Can you work these out from the model? Positions are in its coordinate system, mm. Face numbers are marked on the shaded views. A direction names the side the tool comes from. Give positions to 0.01 mm unless a question says otherwise; leave off trailing zeros. Order: outer loops, then holes, each group sorted by start corner. A loop starts at its lowest first (then second) coordinate and runs counter-clockwise, first axis right, second up. Notation, with made-up numbers: (46, -26.5) - (102, -26.5) arc R9 cw to (102, -11.5) - close; hole circle Ø8 at (18, 48.25). An arc over 180 degrees is marked (long way). Answer as a JSON object with one key per item and string values.
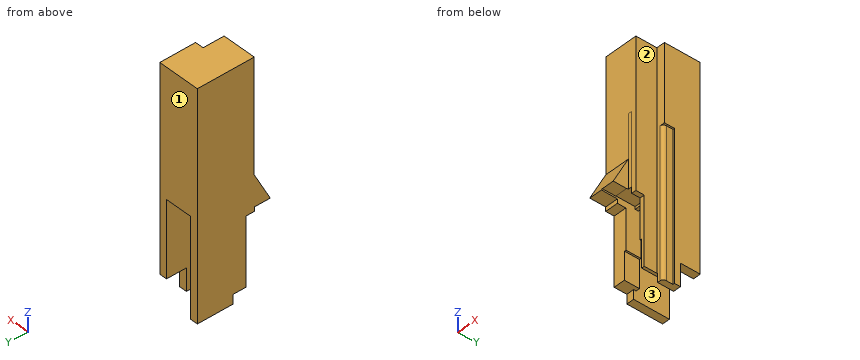
```python
from build123d import *

# Parameters (mm, degrees)
SKETCH1_W           = 50
SKETCH1_H           = 86.52
BOSS_EXTRUDE1_DEPTH = 266.658
SKETCH2_W           = 32
SKETCH2_H           = 116.66
CUT_EXTRUDE1_DEPTH  = 39.55
SKETCH3_W           = 32
SKETCH3_H           = 11
CUT_EXTRUDE2_DEPTH  = 276.341006506
SKETCH4_W           = 23
SKETCH4_H           = 33
CUT_EXTRUDE3_DEPTH  = 276.341006506
SKETCH5_W           = 19
SKETCH5_H           = 52
CUT_EXTRUDE4_DEPTH  = 276.341006506
SKETCH6_W           = 19
SKETCH6_H           = 3
CUT_EXTRUDE5_DEPTH  = 3
SKETCH7_W           = 26.66
SKETCH7_H           = 23.55
CUT_EXTRUDE6_DEPTH  = 11
SKETCH8_W           = 96.66
SKETCH8_H           = 18.97
CUT_EXTRUDE7_DEPTH  = 285.76692112
SKETCH9_W           = 80.656
SKETCH9_H           = 10
CUT_EXTRUDE8_DEPTH  = 285.76692112
SKETCH10_W          = 11
SKETCH10_H          = 25
CUT_EXTRUDE9_DEPTH  = 285.76692112
SKETCH11_W          = 175.66
SKETCH11_H          = 55.97
CUT_EXTRUDE10_DEPTH = 2
SKETCH12_W          = 266.658
SKETCH12_H          = 59.418393815
CUT_EXTRUDE11_DEPTH = 10
FILLET2_R           = 4
SKETCH13_W          = 19
SKETCH13_H          = 48.117373491
CUT_EXTRUDE12_DEPTH = 2.659
SKETCH16_W          = 19
SKETCH16_H          = 23.032
CUT_EXTRUDE13_DEPTH = 0.341
CUT_EXTRUDE14_DEPTH = 284.182272334
CUT_EXTRUDE15_DEPTH = 10
SKETCH22_W          = 5.5
SKETCH22_H          = 5.004
CUT_EXTRUDE16_DEPTH = 0.03
SKETCH24_W          = 4.5
SKETCH24_H          = 85.486763268
BOSS_EXTRUDE2_DEPTH = 0.03


with BuildPart() as part:
    # Sketch1 → Boss-Extrude1 (new body)
    with BuildSketch(Plane.XY):
        with Locations((-25, 43.26)):
            Rectangle(SKETCH1_W, SKETCH1_H)
    extrude(amount=BOSS_EXTRUDE1_DEPTH)

    # Sketch2 → Cut-Extrude1 (cut)
    with BuildSketch(Plane(origin=(0, 86.52, 0), x_dir=(1, 0, 0), z_dir=(0, 1, 0))):
        with Locations((-25, -58.33)):
            Rectangle(SKETCH2_W, SKETCH2_H)
    extrude(amount=-CUT_EXTRUDE1_DEPTH, mode=Mode.SUBTRACT)

    # Sketch3 → Cut-Extrude2 (cut, through all)
    with BuildSketch(Plane(origin=(0, 46.97, 0), x_dir=(1, 0, 0), z_dir=(0, 1, 0))):
        with Locations((-25, -5.5)):
            Rectangle(SKETCH3_W, SKETCH3_H)
    extrude(amount=-CUT_EXTRUDE2_DEPTH, mode=Mode.SUBTRACT)

    # Sketch4 → Cut-Extrude3 (cut, through all)
    with BuildSketch(Plane(origin=(0, 46.97, 0), x_dir=(1, 0, 0), z_dir=(0, 1, 0))):
        with Locations((-25, -27.5)):
            Rectangle(SKETCH4_W, SKETCH4_H)
    extrude(amount=-CUT_EXTRUDE3_DEPTH, mode=Mode.SUBTRACT)

    # Sketch5 → Cut-Extrude4 (cut, through all)
    with BuildSketch(Plane(origin=(0, 46.97, 0), x_dir=(1, 0, 0), z_dir=(0, 1, 0))):
        with Locations((-25, -70)):
            Rectangle(SKETCH5_W, SKETCH5_H)
    extrude(amount=-CUT_EXTRUDE4_DEPTH, mode=Mode.SUBTRACT)

    # Sketch6 → Cut-Extrude5 (cut)
    with BuildSketch(Plane(origin=(0, 46.97, 0), x_dir=(1, 0, 0), z_dir=(0, 1, 0))):
        with Locations((-25, -97.5)):
            Rectangle(SKETCH6_W, SKETCH6_H)
    extrude(amount=-CUT_EXTRUDE5_DEPTH, mode=Mode.SUBTRACT)

    # Sketch7 → Cut-Extrude6 (cut)
    with BuildSketch(Plane(origin=(0, 0, 0), x_dir=(0, 0, -1), z_dir=(1, 0, 0))):
        with Locations((-13.33, 74.745)):
            Rectangle(SKETCH7_W, SKETCH7_H)
    extrude(amount=-CUT_EXTRUDE6_DEPTH, mode=Mode.SUBTRACT)

    # Sketch8 → Cut-Extrude7 (cut, through all)
    with BuildSketch(Plane(origin=(0, 0, 0), x_dir=(0, 0, -1), z_dir=(1, 0, 0))):
        with Locations((-48.33, 9.485)):
            Rectangle(SKETCH8_W, SKETCH8_H)
    extrude(amount=-CUT_EXTRUDE7_DEPTH, mode=Mode.SUBTRACT)

    # Sketch9 → Cut-Extrude8 (cut, through all)
    with BuildSketch(Plane(origin=(0, 0, 0), x_dir=(0, 0, -1), z_dir=(1, 0, 0))):
        with Locations((-51.328, 23.97)):
            Rectangle(SKETCH9_W, SKETCH9_H)
    extrude(amount=-CUT_EXTRUDE8_DEPTH, mode=Mode.SUBTRACT)

    # Sketch10 → Cut-Extrude9 (cut, through all)
    with BuildSketch(Plane(origin=(0, 0, 0), x_dir=(0, 0, -1), z_dir=(1, 0, 0))):
        with Locations((-5.5, 31.47)):
            Rectangle(SKETCH10_W, SKETCH10_H)
    extrude(amount=-CUT_EXTRUDE9_DEPTH, mode=Mode.SUBTRACT)

    # Sketch11 → Cut-Extrude10 (cut)
    with BuildSketch(Plane(origin=(0, 0, 0), x_dir=(0, 0, -1), z_dir=(1, 0, 0))):
        with Locations((-87.83, 27.985)):
            Rectangle(SKETCH11_W, SKETCH11_H)
    extrude(amount=-CUT_EXTRUDE10_DEPTH, mode=Mode.SUBTRACT)

    # Sketch12 → Cut-Extrude11 (cut)
    with BuildSketch(Plane(origin=(0, 0, 0), x_dir=(0, 0, -1), z_dir=(1, 0, 0))):
        with Locations((-133.329, 14.260803093)):
            Rectangle(SKETCH12_W, SKETCH12_H)
    extrude(amount=-CUT_EXTRUDE11_DEPTH, mode=Mode.SUBTRACT)

    # Fillet2
    fillet2_edges = [part.edges().sort_by_distance(p)[0] for p in [
        (-2, 43.97, 87.83),
    ]]
    fillet(fillet2_edges, radius=FILLET2_R)

    # Sketch13 → Cut-Extrude12 (cut)
    with BuildSketch(Plane(origin=(0, 0, 96), x_dir=(-1, 0, 0), z_dir=(0, 0, -1))):
        with Locations((25, 15.911313255)):
            Rectangle(SKETCH13_W, SKETCH13_H)
    extrude(amount=-CUT_EXTRUDE12_DEPTH, mode=Mode.SUBTRACT)

    # Sketch16 → Cut-Extrude13 (cut)
    with BuildSketch(Plane(origin=(0, 0, 98.659), x_dir=(-1, 0, 0), z_dir=(0, 0, -1))):
        with Locations((25, 28.454)):
            Rectangle(SKETCH16_W, SKETCH16_H)
    extrude(amount=-CUT_EXTRUDE13_DEPTH, mode=Mode.SUBTRACT)

    # Sketch18 → Cut-Extrude14 (cut, through all)
    with BuildSketch(Plane(origin=(-10, 0, 0), x_dir=(0, 0, -1), z_dir=(1, 0, 0))):
        Polygon((-133.131, 19), (-96.66, 0), (-266.658, 0), (-266.658, 19), align=None)
    extrude(amount=-CUT_EXTRUDE14_DEPTH, mode=Mode.SUBTRACT)

    # Sketch19 → Cut-Extrude15 (cut)
    with BuildSketch(Plane(origin=(-10, 0, 0), x_dir=(0, 0, -1), z_dir=(1, 0, 0))):
        Polygon((-96.66, 0), (-133.131, 19), (-96.66, 19), align=None)
    extrude(amount=-CUT_EXTRUDE15_DEPTH, mode=Mode.SUBTRACT)

    # Sketch22 → Cut-Extrude16 (cut)
    with BuildSketch(Plane.XZ.offset(-18.97)):
        with Locations((-12.75, 94.158)):
            Rectangle(SKETCH22_W, SKETCH22_H)
    extrude(amount=-CUT_EXTRUDE16_DEPTH, mode=Mode.SUBTRACT)

    # Sketch24 → Boss-Extrude2 (add)
    with BuildSketch(Plane.XZ.offset(-19)):
        with Locations((-17.75, 141.743381634)):
            Rectangle(SKETCH24_W, SKETCH24_H)
    extrude(amount=BOSS_EXTRUDE2_DEPTH)


solid = part.part
```
Q1. I'm going to push flat-ended pins straight in: pin 1 Ø0.9 at (x, z) = (-20.5, 97.5) entering from -Y; pin 2 Ø5.5 at (y, z) = (35, 27.5) entering from +X; pin 3 Ø1.5 at (x, z) = (-43, 95) entering from -Y. Where does each tip first touch, or does it pass through?
Recorded:
{"pin 1": "stops at y = 39.97", "pin 2": "stops at x = -10", "pin 3": "stops at y = 18.97"}
Q2. I need wall thicknesses on L1, parallel to X at y = 49, z = 62; L2, parallel to Z at x = -39.5, y = 41; L3, parallel to Y at x = -8.5, z = 67. Which ranges of each line are inside material? Lowest first, please.
Recorded:
{"L1": "x = -50 to -41, -9 to -2", "L2": "z = 11 to 266.66", "L3": "y = 43.97 to 86.52"}
Q3. If we section it at C-C, the plane y = 78: Please give me the cut outline in (x, z), then the cut area to 3 significant figures.
Recorded:
{"outline": "(-50, 0) - (-41, 0) - (-41, 116.66) - (-9, 116.66) - (-9, 26.66) - (0, 26.66) - (0, 266.66) - (-50, 266.66) - close", "area": "9,360 mm^2"}
Q4. Which directions (+Z, -Z, +X, -X, +Y, -Y) give clear straight access to the entire face, cutting with the end or side of a thin tool? Please do the marked faces 1, 2 and 3.
Recorded:
{"face 1": "+Z, -Z, +X, -X, +Y", "face 2": "+Z, -Z, +X, -Y", "face 3": "-Z, +Y"}
Q5. If we section it at B-B, the plane x = -47: Please give me the cut outline in (y, z).
Recorded:
{"outline": "(0, 96.66) - (18.97, 96.66) - (18.97, 91.66) - (28.97, 91.66) - (28.97, 11) - (43.97, 11) - (43.97, 0) - (86.52, 0) - (86.52, 266.66) - (19, 266.66) - (19, 133.13) - close"}
Q6. If we section it at A-A, the plane z = 67.5: Please give me the cut outline in (x, y).
Recorded:
{"outline": "(-50, 28.97) - (-34.5, 28.97) - (-34.5, 46.97) - (-41, 46.97) - (-41, 86.52) - (-50, 86.52) - close; (-15.5, 28.97) - (-10, 28.97) - (-10, 43.97) - (-6, 43.97) arc R4 ccw to (-2, 47.97) - (-2, 55.97) - (0, 55.97) - (0, 86.52) - (-9, 86.52) - (-9, 46.97) - (-15.5, 46.97) - close"}
